Source: CAD feature listing. Evaluate the final solid. Frame: model axes, mm. Face numbers are marked on the shaded views. Coordinates: 2 decimals unless noted, no trailing zeros. Order: outer loops, then holes, each group sorted by start corner. A loop starts at its lowest first (then second) coordinate and runs counter-clockwise, first axis right, second up.
```python
from build123d import *

# Parameters (mm, degrees)
BOSS_EXTRUDE1_DEPTH = 67.3735
SKETCH2_R           = 5.0292
BOSS_EXTRUDE2_DEPTH = 1.1684
BOSS_EXTRUDE3_DEPTH = 2.54
BOSS_EXTRUDE4_START = 1.1684
SKETCH5_R           = 5.0292
BOSS_EXTRUDE4_DEPTH = 1.1684
BOSS_EXTRUDE5_DEPTH = 2.54


with BuildPart() as part:
    # Sketch1 → Boss-Extrude1 (new body)
    with BuildSketch(Plane.XY):
        Polygon((5.908332382, -4.342227746), (6.714645728, 2.945652064), (0.806313346, 7.28787981), (-5.908332382, 4.342227746), (-6.714645728, -2.945652064), (-0.806313346, -7.28787981), align=None)
    extrude(amount=BOSS_EXTRUDE1_DEPTH)

    # Sketch2 → Boss-Extrude2 (add)
    with BuildSketch(Plane.XY.offset(67.3735)):
        Circle(SKETCH2_R)
    extrude(amount=BOSS_EXTRUDE2_DEPTH)

    # Sketch3 → Boss-Extrude3 (add)
    with BuildSketch(Plane.XY.offset(68.5419)):
        Polygon((-0.806313346, -7.28787981), (5.908332382, -4.342227746), (6.714645728, 2.945652064), (0.806313346, 7.28787981), (-5.908332382, 4.342227746), (-6.714645728, -2.945652064), align=None)
    extrude(amount=BOSS_EXTRUDE3_DEPTH)

    # Sketch5 → Boss-Extrude4 (add)
    with BuildSketch(Plane(origin=(0, 0, 0), x_dir=(-1, 0, 0), z_dir=(0, 0, -1)).offset(BOSS_EXTRUDE4_START)):
        with Locations(Location((0, 0, 0), (0, 0, 180))):
            Circle(SKETCH5_R)
    extrude(amount=-BOSS_EXTRUDE4_DEPTH)

    # Sketch6 → Boss-Extrude5 (add)
    with BuildSketch(Plane(origin=(0, 0, -1.1684), x_dir=(-1, 0, 0), z_dir=(0, 0, -1))):
        Polygon((-5.908332382, -4.342227746), (0.806313346, -7.28787981), (6.714645728, -2.945652064), (5.908332382, 4.342227746), (-0.806313346, 7.28787981), (-6.714645728, 2.945652064), align=None)
    extrude(amount=BOSS_EXTRUDE5_DEPTH)


solid = part.part
```
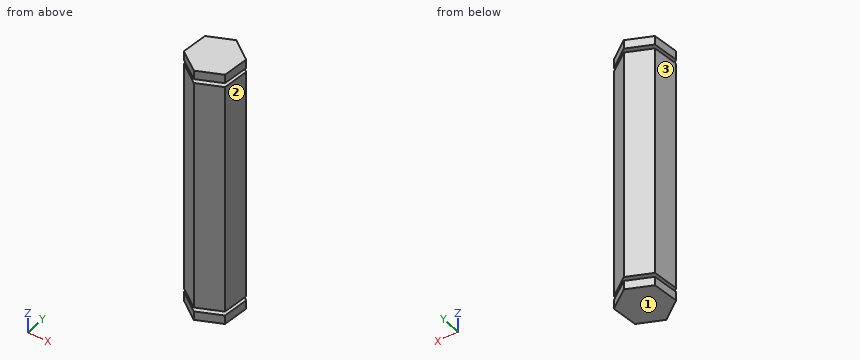
1. Contact query for flat-ended pins moving along their axis: P1, Ø1, axis at y = 0, z = 22.5, coming from the -X side; P2, Ø2, axis at x = -2.5, z = 56, coming from the -Y side; P3, Ø2, axis at x = -3, z = 31, coming from the -Y side. Output: stop coordinate, or through.
2. Section query A-A, the plane z = 21.5. Output: boundary loops of the cut face in (x, y), plus the area to 3 significant figures.
3. Draft query along Y for the marked faces 1, 2 and 3. Return one class per face: +Y half, -Y half, draft (parallel to the pull), parting line (faces both ways), or undercut.
4. Material intervals for line 1 along Z through (x, y) = (0.75, -6.25); line 2 along X through (y, z) = (6.75, 42.5); line 3 along Y through (x, z) = (4.75, 62), sorted ascending.
5. Section query B-B, the plane y = -1. Output: boundary loops of the cut face in (x, z).
6. Section query C-C, the plane x = -1.5. Output: boundary loops of the cut face in (y, z).
Answer key:
1. P1: stops at x = -6.44
1. P2: stops at y = -6.78
1. P3: stops at y = -6.41
2. outline: (-6.71, -2.95) - (-0.81, -7.29) - (5.91, -4.34) - (6.71, 2.95) - (0.81, 7.29) - (-5.91, 4.34) - close
2. area: 140 mm2
3. face 1: draft
3. face 2: -Y half
3. face 3: +Y half
4. line 1: z = -3.71 to -1.17, 0 to 67.37, 68.54 to 71.08
4. line 2: x = -0.42 to 1.54
4. line 3: y = -4.85 to 4.39
5. outline: (-6.5, -3.71) - (6.28, -3.71) - (6.28, -1.17) - (4.93, -1.17) - (4.93, 0) - (6.28, 0) - (6.28, 67.37) - (4.93, 67.37) - (4.93, 68.54) - (6.28, 68.54) - (6.28, 71.08) - (-6.5, 71.08) - (-6.5, 68.54) - (-4.93, 68.54) - (-4.93, 67.37) - (-6.5, 67.37) - (-6.5, 0) - (-4.93, 0) - (-4.93, -1.17) - (-6.5, -1.17) - close
6. outline: (-6.78, -3.71) - (6.28, -3.71) - (6.28, -1.17) - (4.8, -1.17) - (4.8, 0) - (6.28, 0) - (6.28, 67.37) - (4.8, 67.37) - (4.8, 68.54) - (6.28, 68.54) - (6.28, 71.08) - (-6.78, 71.08) - (-6.78, 68.54) - (-4.8, 68.54) - (-4.8, 67.37) - (-6.78, 67.37) - (-6.78, 0) - (-4.8, 0) - (-4.8, -1.17) - (-6.78, -1.17) - close
